```python
from build123d import *

# Parameters (mm, degrees)
SKETCH1_R           = 2.5
BOSS_EXTRUDE1_DEPTH = 2.5


with BuildPart() as part:
    # Sketch1 → Boss-Extrude1 (new body)
    with BuildSketch(Plane(origin=(0, 0, -1.25), x_dir=(-1, 0, 0), z_dir=(0, 0, -1))):
        Polygon((-6.35, -12.7), (50.546, -12.7), (56.896, -6.35), (56.896, 6.35), (50.546, 12.7), (12.7, 12.7), (12.7, 50.546), (6.35, 56.896), (-6.35, 56.896), (-12.7, 50.546), (-12.7, -6.35), align=None)
        with Locations((0, 12.7)):
            Circle(SKETCH1_R, mode=Mode.SUBTRACT)
        with Locations((0, 25.4)):
            Circle(SKETCH1_R, mode=Mode.SUBTRACT)
        with Locations((12.7, 0)):
            Circle(SKETCH1_R, mode=Mode.SUBTRACT)
        with Locations((25.4, 0)):
            Circle(SKETCH1_R, mode=Mode.SUBTRACT)
        Circle(SKETCH1_R, mode=Mode.SUBTRACT)
        with Locations((50.8, 0)):
            Circle(SKETCH1_R, mode=Mode.SUBTRACT)
        with Locations((38.1, 0)):
            Circle(SKETCH1_R, mode=Mode.SUBTRACT)
        with Locations((0, 50.8)):
            Circle(SKETCH1_R, mode=Mode.SUBTRACT)
        with Locations((0, 38.1)):
            Circle(SKETCH1_R, mode=Mode.SUBTRACT)
    extrude(amount=-BOSS_EXTRUDE1_DEPTH)


solid = part.part
```
Could you check a few things on this model? Use its own coordinates, in mm. A direction names the side the tool comes from. Coordinates: 2 decimals unless noted, no trailing zeros. Order: outer loops, then holes, each group sorted by start corner. A loop starts at its lowest first (then second) coordinate and runs counter-clockwise, first axis right, second up. Notation, with made-up numbers: M -30.5,-24 L 20.5,-24 A17 ccw 20.5,-17 Z; hole C -31.75,30 d2. An arc over 180 degrees is marked long. Use a Markdown table: item, result. Add a question column.
Q1. I want a section at A-A on y = 25.4. List the corners of the cut face in (x, z) for me, then the cut area to 3 significant figures.
Q2. Which directions (+Z, -Z, +X, -X, +Y, -Y) give clear straight access to the entire face, cutting with the end or side of a thin tool? Please do faces 4 (the cylindrical face through (0.54, -2.44, -0.02)), 5 (the flat face through (-32, 12.7, 0)).
Q3. I want a section at D-D on y = 42. List the corners of the cut face in (x, z) for me, then the cut area to 3 significant figures.
Q4. I'm going to push a flat-ended pin straight in: pin 1 (0.8 mm diameter, centred on y = 26.5, z = 0, fed in from -X). Where does the tip first touch, or does it pass through?
Q5. I want a section at B-B on z = 0.65. Give the number of separate pieces and of enclosed holes in the cut face, then the cut area to 3 significant figures.
Q6. If I drill on L1, parallel to Y at x = 0, z = 0.6; L2, parallel to X at y = -0.5, z = 0.45; L3, parallel to Y at x = 1.5, z = -0.2, over which ranges is the centre line in solid material (lowest first)?
Q7. We'd pull the mould along X, two halves only. Please class faces 1 (the flat face through (-53.765, 9.481, -0.018)), 2 (the flat face through (9.57, -9.48, -0.02)), 3 (the cylindrical face through (-1.34, 52.91, -0.02)): pulls with the +X half, pulls with the -X half, needs draft (parallel to the pull), parting line crosses it, or undercut.
Checked values:
| question | item | result |
|---|---|---|
| 1 | outline | M -12.7,-1.25 L -2.5,-1.25 L -2.5,1.25 L -12.7,1.25 Z; M 2.5,-1.25 L 12.7,-1.25 L 12.7,1.25 L 2.5,1.25 Z |
| 1 | area | 51.0 mm² |
| 2 | face 4 | +Z, -Z |
| 2 | face 5 | +Z, -Z, -X, +Y |
| 3 | outline | M -12.7,-1.25 L 12.7,-1.25 L 12.7,1.25 L -12.7,1.25 Z |
| 3 | area | 63.5 mm² |
| 4 | pin 1 | x = -12.7 |
| 5 | separate pieces | 1 |
| 5 | enclosed holes | 9 |
| 5 | area | 2,610 mm² |
| 6 | L1 | -12.7 to -2.5, 2.5 to 10.2, 15.2 to 22.9, 27.9 to 35.6, 40.6 to 48.3, 53.3 to 56.9 |
| 6 | L2 | -56.9 to -53.25, -48.35 to -40.55, -35.65 to -27.85, -22.95 to -15.15, -10.25 to -2.45, 2.45 to 12.7 |
| 6 | L3 | -12.7 to -2, 2 to 10.7, 14.7 to 23.4, 27.4 to 36.1, 40.1 to 48.8, 52.8 to 56.9 |
| 7 | face 1 | pulls with the -X half |
| 7 | face 2 | pulls with the +X half |
| 7 | face 3 | undercut |
